The listing builds one solid part. Answer for the finished solid, in the listing's coordinates (mm). A direction names the side the tool comes from. Round coordinates to 2 decimals unless told otherwise and drop trailing zeros. Write each loop counter-clockwise with the first axis right and the second up, starting at its lowest first coordinate (ties: lowest second). Pieces come first, ordered by that corner, then holes. Notation, with made-up numbers: M -22,41.25 L 26,41.25 A28 ccw 26,60.25 Z; hole C -2,87 d8. An arc over 180 degrees is marked long. One line per item, written item: value. Start each with the question number.
(1) Section B-B (x = 15) is taken. Determine the outline of the cut face in (y, z), plus the area to 3 significant figures.
(2) Section C-C (y = -92) is taken. Determine the outline of the cut face in (x, z).
(3) Section A-A (z = 0) is taken. Determine the outline of the cut face in (x, y).
(4) For a pull along X with two mould halves and no side action, classify faces 5 (the flat face through (0, 13, 35)), 6 (the flat face through (-1, 10, 37.5)), 7 (the cylindrical face through (33.47, -54.23, 27.96)) as released by +X, released by -X, zero draft, split by the parting line, or undercut.
(5) Given P1, Ø3.5, axis at x = -29, z = -28, coming from the -Y side; P2, Ø3, axis at x = 6.5, z = 20.5, coming from the -Y side; P3, Ø1, axis at x = -1.5, y = -48.5, coming from the +Z side, each flat-ended and moving along its own axis, determine where each tip first touches the part or whether it passes through.
(6) Section D-D (z = -12) is taken. Determine the outline of the cut face in (x, y).
(7) For faces 1 (the flat face through (8, 0, -9)), 2 (the flat face through (30, -105, 28)), 3 (the flat face through (0, 5, 0)), 4 (the flat face through (0.6, -142, 0)), determine the directions among +Z, -Z, +X, -X, +Y, -Y from which every point of the face is accessible in a straight line to the end or side of a thin tool.
(8) Consider probe 1 along Y at (x, z) = (33, 9); probe 2 along X at (y, z) = (-85, 0); probe 3 along Y at (x, z) = (-2, 8). Determine where each line is inside the solid, lowest interval first.
```python
from build123d import *

# Parameters (mm, degrees)
ESBO_O1_W                = 75
ESBO_O1_H                = 75
RESSALTO_EXTRUS_O1_DEPTH = 20
ESBO_O2_W                = 70
ESBO_O2_H                = 70
CORTE_EXTRUS_O1_DEPTH    = 15
ESBO_O3_R                = 5
RESSALTO_EXTRUS_O2_DEPTH = 148
ESBO_O5_W                = 1.2
ESBO_O5_H                = 7
CORTE_EXTRUS_O2_DEPTH    = 70
ESBO_O7_R                = 3.5
RESSALTO_EXTRUS_O3_DEPTH = 105
FILETE2_R                = 5
FILETE3_R                = 5
FILETE4_R                = 5


with BuildPart() as part:
    # Esboço1 → Ressalto-extrusão1 (new body)
    with BuildSketch(Plane(origin=(0, 0, 0), x_dir=(1, 0, 0), z_dir=(0, 1, 0))):
        Rectangle(ESBO_O1_W, ESBO_O1_H)
    extrude(amount=RESSALTO_EXTRUS_O1_DEPTH)

    # Esboço2 → Corte-extrusão1 (cut)
    with BuildSketch(Plane(origin=(0, 20, 0), x_dir=(1, 0, 0), z_dir=(0, 1, 0))):
        Rectangle(ESBO_O2_W, ESBO_O2_H)
    extrude(amount=-CORTE_EXTRUS_O1_DEPTH, mode=Mode.SUBTRACT)

    # Esboço3 → Ressalto-extrusão2 (add)
    with BuildSketch(Plane(origin=(0, 0, 0), x_dir=(-1, 0, 0), z_dir=(0, -1, 0))):
        with Locations(Location((0, 0, 0), (0, 0, 90))):
            Circle(ESBO_O3_R)
    extrude(amount=RESSALTO_EXTRUS_O2_DEPTH)

    # Esboço5 → Corte-extrusão2 (cut)
    with BuildSketch(Plane(origin=(0, 0, -37.5), x_dir=(-1, 0, 0), z_dir=(0, 0, -1))):
        with Locations((0, -142)):
            Rectangle(ESBO_O5_W, ESBO_O5_H)
    extrude(amount=-CORTE_EXTRUS_O2_DEPTH, mode=Mode.SUBTRACT)

    # Esboço7 → Ressalto-extrusão3 (add)
    with BuildSketch(Plane.XZ):
        with Locations(Location((30, 27.5, 0), (0, 0, 270))):
            Circle(ESBO_O7_R)
        with Locations(Location((-30, -27.5, 0), (0, 0, 270))):
            Circle(ESBO_O7_R)
    extrude(amount=RESSALTO_EXTRUS_O3_DEPTH)

    # Filete2
    filete2_edges = [part.edges().sort_by_distance(p)[0] for p in [
        (-30, 0, -24),
    ]]
    fillet(filete2_edges, radius=FILETE2_R)

    # Filete3
    filete3_edges = [part.edges().sort_by_distance(p)[0] for p in [
        (30, 0, 31),
    ]]
    fillet(filete3_edges, radius=FILETE3_R)

    # Filete4
    filete4_edges = [part.edges().sort_by_distance(p)[0] for p in [
        (0, 0, 5),
    ]]
    fillet(filete4_edges, radius=FILETE4_R)


solid = part.part
```
Recorded:
1. outline: M 0,-37.5 L 20,-37.5 L 20,-35 L 5,-35 L 5,35 L 20,35 L 20,37.5 L 0,37.5 Z
1. area: 450 mm2
2. outline: C -30,-27.5 d7; C 0,0 d10; C 30,27.5 d7
3. outline: M -37.5,0 L -10,0 A5 cw -5,-5 L -5,-148 L 5,-148 L 5,-5 A5 cw 10,0 L 37.5,0 L 37.5,20 L 35,20 L 35,5 L -35,5 L -35,20 L -37.5,20 Z; hole M -0.6,-145.5 L 0.6,-145.5 L 0.6,-138.5 L -0.6,-138.5 Z
4. face 5: undercut
4. face 6: zero draft
4. face 7: split by the parting line
5. P1: stops at y = -105
5. P2: stops at y = 0
5. P3: stops at z = 4.9
6. outline: M -37.5,0 L 37.5,0 L 37.5,20 L 35,20 L 35,5 L -35,5 L -35,20 L -37.5,20 Z
7. face 1: -Y
7. face 2: +Z, -Z, +X, -X, -Y
7. face 3: +Y
7. face 4: +Z, -Z
8. probe 1: y = 0 to 5
8. probe 2: x = -5 to 5
8. probe 3: y = -0.32 to 5
